Input: part model. Units: mm. Frame: model coordinates. Face numbers are marked on the shaded views. A direction names the side the tool comes from. Coordinates: 2 decimals unless noted, no trailing zeros. Write each loop counter-clockwise with the first axis right and the second up, starting at its lowest first coordinate (ties: lowest second). Pieces come first, ordered by that corner, then holes. Notation, with made-up numbers: (-22.75, 3) - (-10.75, 3) arc R21 ccw to (-10.75, 27) - close; hole circle Ø2 at (-26, -34). An arc over 180 degrees is marked (long way). Put each result on its own line as item: value. Start each with the question number.
1. Pin query (flat end, axial travel): pin 1 (10 mm diameter, centred on y = 22, z = 15, fed in from +X); pin 2 (1.5 mm diameter, centred on x = 2.5, z = 9, fed in from +Y); pin 3 (1 mm diameter, centred on x = -1, y = -14.5, fed in from -Z); pin 4 (5 mm diameter, centred on x = -10, y = -11, fed in from +Z). Return the tip coordinate at first contact, or that it passes through.
2. Cut plane D-D, the plane x = -5. Return loops of the section in (y, z).
3. Pull-direction query (Y, two-part tool) for the marked faces 4, 5, 6 and 7; classes: released by +Y, released by -Y, zero draft, split by the parting line, or undercut.
4. Line query: line 1 (X direction, y = 25.5, z = 26); line 2 (Y direction, x = 10.5, z = 26.75); line 3 (X direction, y = 5, z = 12.75). Output: solid intervals per line, ascending.
5. Access query for the marked faces 1, 2 and 3. Directions: +Z, -Z, +X, -X, +Y, -Y. A direction counts if a zero-diameter tool reaches every point of the face in a straight line with its end or side. Return the directions, or none.
6. Cut plane A-A, the plane y = 22. Return loops of the section in (x, z).
7. Cut plane B-B, the plane z = 15. Return loops of the section in (x, y).
8. Cut plane C-C, the plane z = 26.5. Return loops of the section in (x, y).
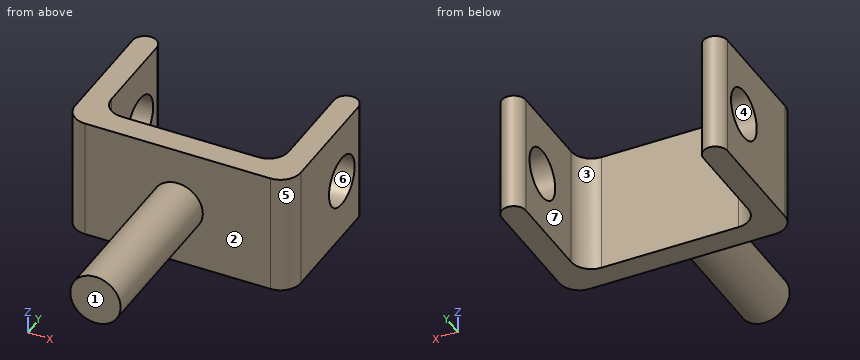
from build123d import *

# Parameters (mm, degrees)
BOSS_EXTRUDE1_DEPTH = 30
SKETCH3_R           = 6.25
BOSS_EXTRUDE2_DEPTH = 40
FILLET1_R           = 5
FILLET2_R           = 5
SKETCH4_R           = 6.25
CUT_EXTRUDE2_DEPTH  = 60


with BuildPart() as part:
    # Sketch2 → Boss-Extrude1 (new body)
    with BuildSketch(Plane.XY):
        with BuildLine():
            Line((-31.831168831, 30), (-31.831168831, -3))
            Line((-31.831168831, -3), (24.168831169, -3))
            Line((24.168831169, -3), (24.168831169, 30))
            ThreePointArc((24.168831169, 30), (21.168831169, 33), (18.168831169, 30))
            Line((18.168831169, 30), (18.168831169, 3))
            Line((18.168831169, 3), (-25.831168831, 3))
            Line((-25.831168831, 3), (-25.831168831, 30))
            ThreePointArc((-25.831168831, 30), (-28.831168831, 33), (-31.831168831, 30))
        make_face()
    extrude(amount=BOSS_EXTRUDE1_DEPTH)

    # Sketch3 → Boss-Extrude2 (add)
    with BuildSketch(Plane.XZ.offset(3)):
        with Locations(Location((-3.831168831, 15, 0), (0, 0, 270))):
            Circle(SKETCH3_R)
    extrude(amount=BOSS_EXTRUDE2_DEPTH)

    # Fillet1
    fillet1_edges = [part.edges().sort_by_distance(p)[0] for p in [
        (-31.831168831, -3, 15),
    ]]
    fillet(fillet1_edges, radius=FILLET1_R)

    # Fillet2
    fillet2_edges = [part.edges().sort_by_distance(p)[0] for p in [
        (24.168831169, -3, 15),
        (-25.831168831, 3, 15),
        (18.168831169, 3, 15),
    ]]
    fillet(fillet2_edges, radius=FILLET2_R)

    # Sketch4 → Cut-Extrude2 (cut)
    with BuildSketch(Plane.ZY.offset(31.831168831)):
        with Locations((15, 22)):
            Circle(SKETCH4_R)
    extrude(amount=-CUT_EXTRUDE2_DEPTH, mode=Mode.SUBTRACT)


solid = part.part
Report:
1. pin 1: passes through
1. pin 2: stops at y = 3
1. pin 3: stops at z = 9.2
1. pin 4: stops at z = 20.06
2. outline: (-43, 8.86) - (-3, 8.86) - (-3, 0) - (3, 0) - (3, 30) - (-3, 30) - (-3, 21.14) - (-43, 21.14) - close
3. face 4: undercut
3. face 5: released by -Y
3. face 6: undercut
3. face 7: zero draft
4. line 1: x = -31.83 to -25.83, 18.17 to 24.17
4. line 2: y = -3 to 3
4. line 3: x = -31.83 to -24.83, 17.17 to 24.17
5. face 1: +Z, -Z, +X, -X, -Y
5. face 2: -Y
5. face 3: +Z, -Z, +Y
6. outline: (-31.83, 0) - (-25.83, 0) - (-25.83, 8.75) - (-31.83, 8.75) - close; (-31.83, 21.25) - (-25.83, 21.25) - (-25.83, 30) - (-31.83, 30) - close; (18.17, 0) - (24.17, 0) - (24.17, 8.75) - (18.17, 8.75) - close; (18.17, 21.25) - (24.17, 21.25) - (24.17, 30) - (18.17, 30) - close
7. outline: (-31.83, 2) arc R5 ccw to (-26.83, -3) - (-10.08, -3) - (-10.08, -43) - (2.42, -43) - (2.42, -3) - (19.17, -3) arc R5 ccw to (24.17, 2) - (24.17, 15.75) - (18.17, 15.75) - (18.17, 8) arc R5 cw to (13.17, 3) - (-20.83, 3) arc R5 cw to (-25.83, 8) - (-25.83, 15.75) - (-31.83, 15.75) - close; (-31.83, 28.25) - (-25.83, 28.25) - (-25.83, 30) arc R3 ccw to (-31.83, 30) - close; (18.17, 28.25) - (24.17, 28.25) - (24.17, 30) arc R3 ccw to (18.17, 30) - close
8. outline: (-31.83, 2) arc R5 ccw to (-26.83, -3) - (19.17, -3) arc R5 ccw to (24.17, 2) - (24.17, 30) arc R3 ccw to (18.17, 30) - (18.17, 8) arc R5 cw to (13.17, 3) - (-20.83, 3) arc R5 cw to (-25.83, 8) - (-25.83, 30) arc R3 ccw to (-31.83, 30) - close
